The drawing under review shows one solid part. Ordinate dimensions are in mm from its lowest x, y, z. Round coordinates to 2 decimals unless told otherwise and drop trailing zeros. Write each loop counter-clockwise with the first axis right and the second up, starting at its lowest first coordinate (ties: lowest second). Pieces come first, ordered by that corner, then holes. Notation, with made-up numbers: (-32.75, 10) -> (-20.75, 10) arc R22 ccw to (-20.75, 43) -> close; hole circle Ø11 at (55, 31.25). An arc over 180 degrees is marked (long way). Write item = value, one per line. Start each with the question number.
Item 1: Add section C-C, the plane x = 57.15. State the section outline as (y, z) points, then the cut area to 3 significant figures.
Item 2: Add section B-B, the plane y = 36.83. State how many separate pieces and enclosed holes the cut face has, then the cut area to 3 significant figures.
Item 3: Add section D-D, the plane z = 17. State the section outline as (x, y) points, then the cut area to 3 significant figures.
Item 4: To check wall thickness, follow L1, parallel to X at y = 11.5, z = 12.5 (1 decimal); L2, parallel to X at y = 23.5, z = 5.75 (1 decimal); L3, parallel to X at y = 15.5, z = 8 (1 decimal). State the ranges of each line that lie inside material, in increasing order.
Item 5: Mouldability with a two-part tool opening along Z and no side actions: class the marked faces 1, 2 and 3 as released by +Z, released by -Z, zero draft, split by the parting line, or undercut.
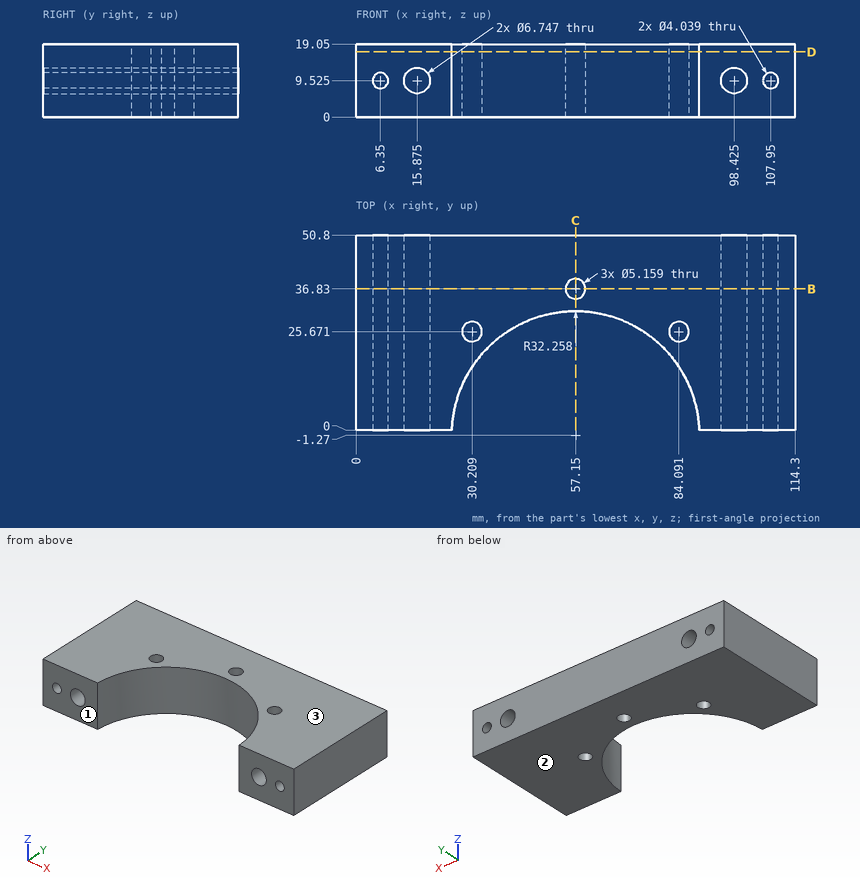
Result set:
q1.outline = (30.99, 0) -> (34.25, 0) -> (34.25, 19.05) -> (30.99, 19.05) -> close; (39.41, 0) -> (50.8, 0) -> (50.8, 19.05) -> (39.41, 19.05) -> close
q1.area = 279 mm²
q2.separate_pieces = 2
q2.enclosed_holes = 4
q2.area = 1,980 mm²
q3.outline = (0, 0) -> (24.92, 0) arc R32.26 cw to (89.38, 0) -> (114.3, 0) -> (114.3, 50.8) -> (0, 50.8) -> close; hole circle Ø5.16 at (30.21, 25.67); hole circle Ø5.16 at (57.15, 36.83); hole circle Ø5.16 at (84.09, 25.67)
q3.area = 4,190 mm²
q4.L1 = 0 to 14.3, 17.5 to 27.5, 86.8 to 96.8, 100 to 114.3
q4.L2 = 0 to 28.8, 31.6 to 36.5, 77.8 to 82.7, 85.5 to 114.3
q4.L3 = 0 to 5, 7.7 to 12.9, 18.9 to 29.6, 84.7 to 95.4, 101.4 to 106.6, 109.3 to 114.3
q5.face_1 = zero draft
q5.face_2 = released by -Z
q5.face_3 = released by +Z
